```python
from build123d import *

# Parameters (mm, degrees)
SKETCH2_R           = 30
SKETCH2_R_2         = 15
BOSS_EXTRUDE1_DEPTH = 25
BOSS_EXTRUDE2_DEPTH = 5
SKETCH4_R           = 6
BOSS_EXTRUDE3_DEPTH = 36
SKETCH5_W           = 15
SKETCH5_H           = 7
CUT_EXTRUDE1_DEPTH  = 36


with BuildPart() as part:
    # Sketch2 → Boss-Extrude1 (new body, symmetric)
    with BuildSketch(Plane.XY):
        Circle(SKETCH2_R)
        Circle(SKETCH2_R_2, mode=Mode.SUBTRACT)
    extrude(amount=BOSS_EXTRUDE1_DEPTH, both=True)

    # Sketch3 → Boss-Extrude2 (add, symmetric)
    with BuildSketch(Plane.XY):
        with BuildLine():
            Line((113.533737607, 0), (113.533737607, 18))
            Line((113.533737607, 18), (88.533737607, 18))
            Line((88.533737607, 18), (6.995589774, 29.172962203))
            ThreePointArc((6.995589774, 29.172962203), (29.999485022, 0.175779521), (7.336970855, -29.08898174))
            Line((7.336970855, -29.08898174), (88.533737607, -18))
            Line((88.533737607, -18), (113.533737607, -18))
            Line((113.533737607, -18), (113.533737607, 0))
        make_face()
    extrude(amount=BOSS_EXTRUDE2_DEPTH, both=True)

    # Sketch4 → Boss-Extrude3 (add)
    with BuildSketch(Plane(origin=(0, 18, 0), x_dir=(1, 0, 0), z_dir=(0, 1, 0))):
        with BuildLine():
            Line((88.533737607, 20), (88.533737607, 5))
            Line((88.533737607, 5), (113.533737607, 5))
            Line((113.533737607, 5), (113.533737607, 20))
            ThreePointArc((113.533737607, 20), (101.033737607, 32.5), (88.533737607, 20))
        make_face()
        with Locations(Location((101.033737607, 20, 0), (0, 0, 180))):  # turned: the seam where the file's is
            Circle(SKETCH4_R, mode=Mode.SUBTRACT)
    extrude(amount=-BOSS_EXTRUDE3_DEPTH)

    # Sketch5 → Cut-Extrude1 (cut)
    with BuildSketch(Plane(origin=(113.533737607, 0, 0), x_dir=(0, 0, -1), z_dir=(1, 0, 0))):
        with Locations((12.5, -3.5)):
            Rectangle(SKETCH5_W, SKETCH5_H)
        with Locations((12.5, 3.5)):
            Rectangle(SKETCH5_W, SKETCH5_H)
        Polygon((20, 7), (20, 0), (31.178860048, 0), (40, 0), (40, 7), align=None)
        Polygon((31.178860048, 0), (20, 0), (20, -7), (40, -7), (40, 0), align=None)
    extrude(amount=-CUT_EXTRUDE1_DEPTH, mode=Mode.SUBTRACT)


solid = part.part
```
Check sheet for the modelled part. Datum: model origin and axes. Units: mm. A direction names the side the tool comes from. Give positions to 0.01 mm unless a question says otherwise; leave off trailing zeros. Loops run counter-clockwise (first coordinate to the right, second up) from the corner with the lowest first, then second, coordinate; pieces in that order, holes last. Notation, with made-up numbers: M -12.75,73 L 38.25,73 A17 ccw 38.25,78 Z; hole C 41,66.5 d5. An arc over 180 degrees is marked long. Answer in a Markdown table with one row per item.
1) Cross-section at B-B (z = 1). Enter the section's corners in (x, y).
Solutions:
| item | result |
|---|---|
| outline | M 7,29.17 A30 ccw long 7.34,-29.09 L 88.53,-18 L 113.53,-18 L 113.53,18 L 88.53,18 Z; hole C 0,0 d30 |
2) Mould release check, pull along Z, two halves, no side actions. Record for faces 4 (the face through (60, 0, 5)), 5 (the face through (60, 0, -5)), 6 (the face through (95.31, 12.58, -18.2)), 7 (the face through (95.31, -12.42, -18.2)): released by +Z, released by -Z, zero draft, split by the parting line, or undercut.
Solutions:
| item | result |
|---|---|
| face 4 | released by +Z |
| face 5 | released by -Z |
| face 6 | undercut |
| face 7 | undercut |
3) Tool access check on faces 1 (the face through (88.534, -12, -13)), 2 (the face through (6, 14, -25)), 3 (the face through (-29.97, 1.32, 0.35)). Record the directions out of +Z, -Z, +X, -X, +Y, -Y that give a thin tool (end or side, any length) a straight path to the whole face; none if there is none.
Solutions:
| item | result |
|---|---|
| face 1 | -Z, +Y, -Y |
| face 2 | -Z, -X, +Y, -Y |
| face 3 | none |
4) Cross-section at D-D (z = -28.5). Enter the section's corners in (x, y), plus the area to 3 significant figures.
Solutions:
| item | result |
|---|---|
| outline | M 91.87,-18 L 110.2,-18 L 110.2,-7 L 91.87,-7 Z; M 91.87,7 L 110.2,7 L 110.2,18 L 91.87,18 Z |
| area | 403 mm^2 |
5) Thickness scan on line 1 (Y direction, x = 0, z = -13.5); line 2 (X direction, y = 10.5, z = -22.5); line 3 (Z direction, x = 81.5, y = -14). Record the ranges inside material, lowest first.
Solutions:
| item | result |
|---|---|
| line 1 | y = -30 to -15, 15 to 30 |
| line 2 | x = -28.1 to -10.71, 10.71 to 28.1, 88.79 to 95.58, 106.49 to 113.28 |
| line 3 | z = -5 to 5 |
6) Depth check by flat-ended pin: pin 1 (4 mm diameter, centred on y = -15.5, z = -4.5, fed in from -X); pin 2 (4 mm diameter, centred on x = -3, z = 8.5, fed in from -Y); pin 3 (17.5 mm diameter, centred on x = 45, y = -10, fed in from -Z). Enter the tip coordinate at first touch or a pass-through.
Solutions:
| item | result |
|---|---|
| pin 1 | stops at x = -26.79 |
| pin 2 | stops at y = -29.98 |
| pin 3 | stops at z = -5 |
7) Cross-section at A-A (y = 0). Enter the section's corners in (x, z).
Solutions:
| item | result |
|---|---|
| outline | M -30,-25 L -15,-25 L -15,25 L -30,25 Z; M 15,-25 L 30,-25 L 30,-5 L 113.53,-5 L 113.53,5 L 30,5 L 30,25 L 15,25 Z |
8) Cross-section at C-C (x = 0). Enter the section's corners in (y, z).
Solutions:
| item | result |
|---|---|
| outline | M -30,-25 L -15,-25 L -15,25 L -30,25 Z; M 15,-25 L 30,-25 L 30,25 L 15,25 Z |
